Here's how the part is built. I have some questions about the finished solid (model axes, mm). Face numbers are marked on the shaded views. A direction names the side the tool comes from. Coordinates: 2 decimals unless noted, no trailing zeros. Write each loop counter-clockwise with the first axis right and the second up, starting at its lowest first coordinate (ties: lowest second). Pieces come first, ordered by that corner, then holes.
Item 1: For the marked faces 1 and 2, which set-ups out of +Z, -Z, +X, -X, +Y, -Y let a thin tool reach every point of the face, with its end or its side?
Item 2: Please list where these lines run through material, in increasing order: line 1 (X direction, y = -1.5, z = 8.25); line 2 (Y direction, x = 24, z = -4); line 3 (Y direction, x = 36, z = 5.75).
Item 3: I'm going to push flat-ended pins straight in: P1, Ø3, axis at y = 8.5, z = -6, coming from the +X side; P2, Ø1, axis at x = 45.5, z = 6, coming from the +Y side; P3, Ø10, axis at x = 15, y = 3, coming from the +Z side. Where does each tip first touch, or does it pass through?
Item 4: I want a section at A-A (x = 77). Please give me the cut outline in (y, z), and give its area (3 significant figures).
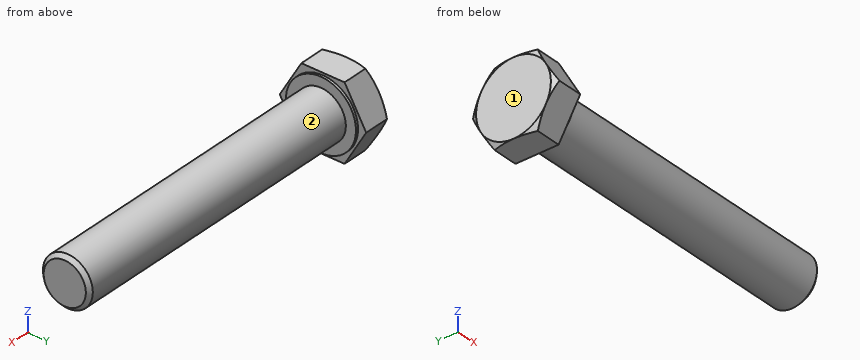
Autodesk Inventor part; units mm, degrees
ref_plane "Work Plane1" through (1.525, 0, 0) normal (0, 0, 1) x (1, 0, 0)
ref_plane "YZ Plane" through (0, 0, 0) normal (1, 0, 0) x (0, 1, 0)
ref_plane "XZ Plane" through (0, 0, 0) normal (0, 1, 0) x (-1, 0, 0)
sketch "Sketch1" plane through (0, 0, 0) normal (0, 0, 1) x (1, 0, 0)
  line L0 (0, 11.245) -> (0, 8)
  line L1 (6, 8) -> (100, 8)
  line L2 (100, 8) -> (100, 0)
  line L3 (100, 0) -> (-0.8001, 0)
  line L4 (-20.9601, 0) -> (120.16, 0)
  line L5 (-0.8001, 0) -> (-0.8001, 11.245)
  line L6 (-0.8001, 11.245) -> (0, 11.245)
  line L7 (6, 8) -> (4.773, 8)
  line L8 (4.773, 8) -> (0, 8)
  line L9 (0, -2.249) -> (0, 13.494)
  dimension "d0" = 100
  dimension "d1" = 94
  dimension "d2" = 16
  dimension "d9" = 0.8001
  dimension "d10" = 22.49
  dimension "d13" = 1.227
  dimension "d14" = 16
revolve "Body" add sketch "Sketch1" angle 360 about axis through (100, 0, 0) along (-1, 0, 0)
sketch "Sketch2" plane through (-0.8001, 0, 0) normal (-1, 0, 0) x (0, 0, 1)
  line L0 (0, 13.8564) -> (12, 6.9282)
  line L1 (12, 6.9282) -> (12, -6.9282)
  line L2 (12, -6.9282) -> (0, -13.8564)
  line L3 (0, -13.8564) -> (-12, -6.9282)
  line L4 (-12, -6.9282) -> (-12, 6.9282)
  line L5 (-12, 6.9282) -> (0, 13.8564)
  point P0 (0, 0)
  point P1 (0, 0)
  dimension "d11" = 24
extrude "Head" add sketch "Sketch2" along normal blind 9.2
sketch "Sketch4" plane through (0, 0, 0) normal (0, 0, 1) x (1, 0, 0)
  line L0 (-10.0001, 12) -> (-10.0001, 13.8564)
  line L1 (-10.0001, 13.8564) -> (-8.9283, 13.8564)
  line L2 (-8.9283, 13.8564) -> (-10.0001, 12)
  line L3 (-11.8401, 0) -> (1.0399, 0)
  line L4 (-0.8001, 13.8564) -> (-10.0001, 13.8564)
  line L5 (-10.0001, 6.9282) -> (-10.0001, 13.8564)
  dimension "d5" = 30
  dimension "d19" = 24
revolve "Chamfer1" cut sketch "Sketch4" angle 360 about axis through (-10, 0, 0) along (1, 0, 0)
thread "Thread"
chamfer "Chamfer2" distance 1.2269 distance2 1.227 1 edges at (100, -8, 0) measured on face at (100, -0.9456, 1.8959)
ref_plane "Work Plane1" through (1.525, 0, 0) normal (0, 0, 1) x (1, 0, 0)
equation "\"d0\" = NLG"
equation "\"d1\" = GEL"
equation "\"d2\" = GD"
equation "\"d10\" = SD2"
equation "\"d14\" = BDM"
equation "\"d11\" = SW"
equation "\"d3\" = KOH - SD"
equation "\"d5\" = ANG1"
equation "\"d19\" = SW0"
equation "\"d15\" = GEL"
equation "\"d6\" = -0.5 * SPD + 0.5 * GD"
equation "\"NLG\" = 100"
equation "\"GD\" = NND"
equation "\"BDM\" = NND"
equation "\"KOH\" = 10"
equation "\"GEL\" = 94"
equation "\"SW\" = 24"
equation "\"SW0\" = SW"
equation "\"SPD\" = NND - 1.2269 * PTC"
equation "\"SD2\" = 22.49"
equation "\"SD\" = 0.8"
equation "\"ANG1\" = 30deg"
equation "\"GAL\" = 0.61345 * PTC"
equation "\"GUL\" = 0.61345 * PTC"
equation "\"RR\" = 0.6"
equation "\"GD1\" = THREADDIA - 1.2269 * PTC"
equation "\"THREADDIA\" = 16"
equation "\"SDH\" = SD2"
equation "\"SDHG\" = 6"
equation "\"TOA\" = 30deg"
equation "\"PTC\" = 2"
equation "\"NND\" = 16"
equation "\"E0\" = 27.72"
properties part number "ISO 4017 - M16 x 100" material "Steel, Mild"
Answer:
1. face 1: +Z, -Z, -X, +Y, -Y
1. face 2: +X
2. line 1: x = -10 to 0
2. line 2: y = -6.93 to 6.93
2. line 3: y = -5.56 to 5.56
3. P1: stops at x = 0
3. P2: stops at y = 5.81
3. P3: stops at z = 8
4. outline: circle Ø16 at (0, 0)
4. area: 201 mm2
